Can you work these out from the model? Positions are in its coordinate system, mm. Round coordinates to 2 decimals unless told otherwise and drop trailing zeros. Return JSON: item names as keys, results as strings.
```python
from build123d import *

# Parameters (mm, degrees)
SKETCH_1_W                  = 95
SKETCH_1_H                  = 830
EXTRUDE_1_DEPTH             = 5
HOLE_WIZARD_1_D             = 6.6
HOLE_WIZARD_1_CBORE_D       = 11
HOLE_WIZARD_1_CBORE_DEPTH   = 6.8
HOLE_WIZARD_M8_1_D          = 6.8
HOLE_WIZARD_M8_2_D          = 6.8
HOLE_WIZARD_2_D             = 6.6
HOLE_WIZARD_2_DEPTH         = 10.001
HOLE_WIZARD_2_CBORE_D       = 11
HOLE_WIZARD_2_CBORE_DEPTH   = 6.8
HOLE_WIZARD_M5_1_D          = 4.2
HOLE_WIZARD_1_2_D           = 9
HOLE_WIZARD_1_2_CSINK_D     = 17.6
HOLE_WIZARD_1_2_CSINK_ANGLE = 90


with BuildPart() as part:
    # 草图1 → 凸台-拉伸1 (new body, symmetric)
    with BuildSketch(Plane.XY):
        Rectangle(SKETCH_1_W, SKETCH_1_H)
    extrude(amount=EXTRUDE_1_DEPTH, both=True)

    # Hole Wizard 1 (through all)
    with Locations(Plane(origin=(-20, -365, 5), x_dir=(1, 0, 0), z_dir=(0, 0, 1))):
        with Locations((0, 0), (40, 0), (40, -40), (0, -40), (0, 385), (40, 385), (40, 345), (0, 345), (0, 770), (40, 770), (40, 730), (0, 730)):
            CounterBoreHole(HOLE_WIZARD_1_D / 2, HOLE_WIZARD_1_CBORE_D / 2, HOLE_WIZARD_1_CBORE_DEPTH)

    # M8 螺纹孔1 (through all)
    with Locations(Plane(origin=(0, -400, 5), x_dir=(1, 0, 0), z_dir=(0, 0, 1))):
        with Locations((0, 0), (0, 130)):
            Hole(HOLE_WIZARD_M8_1_D / 2)

    # M8 螺纹孔2 (through all)
    with Locations(Plane(origin=(0, 280, 5), x_dir=(1, 0, 0), z_dir=(0, 0, 1))):
        with Locations((0, 0), (0, -130)):
            Hole(HOLE_WIZARD_M8_2_D / 2)

    # 打孔尺寸(%根据)内六角圆柱头螺钉的类型2
    with Locations(Plane(origin=(41.5, 400, 5), x_dir=(1, 0, 0), z_dir=(0, 0, 1))):
        with Locations((0, 0), (0, -200), (0, -400), (0, -600), (0, -800)):
            hole_wizard_2 = CounterBoreHole(HOLE_WIZARD_2_D / 2, HOLE_WIZARD_2_CBORE_D / 2, HOLE_WIZARD_2_CBORE_DEPTH, depth=HOLE_WIZARD_2_DEPTH)

    # 镜向1: 打孔尺寸(%根据)内六角圆柱头螺钉的类型2 across plane
    add(hole_wizard_2.mirror(Plane(origin=(0, 0, 0), x_dir=(0, 0, 1), z_dir=(1, 0, 0))), mode=Mode.SUBTRACT)

    # M5 螺纹孔1 (through all)
    with Locations(Plane(origin=(0, 395, 5), x_dir=(1, 0, 0), z_dir=(0, 0, 1))):
        with Locations((0, 0), (0, -40)):
            Hole(HOLE_WIZARD_M5_1_D / 2)

    # Hole Wizard 1 2 (through all)
    with Locations(Plane(origin=(-32.5, 24.75, 5), x_dir=(1, 0, 0), z_dir=(0, 0, 1))):
        with Locations((0, 0), (65, 0), (65, -49.5), (0, -49.5), (0, 359.5), (65, 359.5), (65, 310), (0, 310), (0, -359.5), (65, -359.5), (65, -409), (0, -409)):
            CounterSinkHole(HOLE_WIZARD_1_2_D / 2, HOLE_WIZARD_1_2_CSINK_D / 2, counter_sink_angle=HOLE_WIZARD_1_2_CSINK_ANGLE)


solid = part.part
```
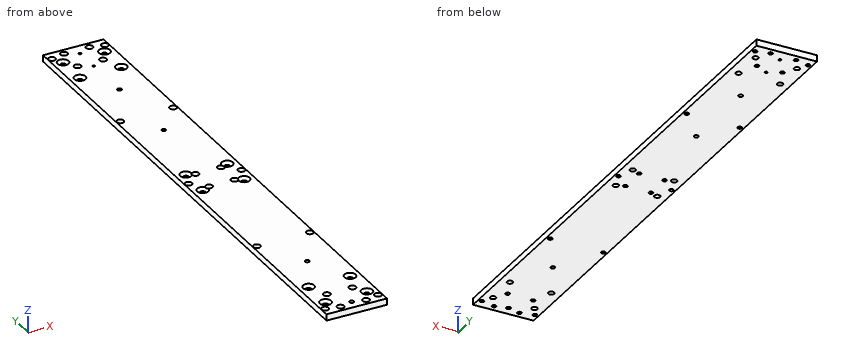
Q1. If I drill on line 1 along X through (y, z) = (203.5, 0); line 2 along X through (y, z) = (29, 3.5), over which ranges is the centre line in solid material (lowest first)?
Results:
{"line 1": "x = -47.5 to -45.74, -37.26 to 37.26, 45.74 to 47.5", "line 2": "x = -47.5 to -38.44, -26.56 to 26.56, 38.44 to 47.5"}
Q2. I'm going to push flat-ended pins straight in: pin 1 Ø9 at (x, y) = (-22, 404) entering from +Z; pin 2 Ø9 at (x, y) = (-41.5, 400) entering from +Z. Where does each tip first touch, or does it pass through?
Results:
{"pin 1": "stops at z = 5", "pin 2": "stops at z = -1.8"}
Q3. Suppose I cut it at A-A, the plane z = 2.75. State how many separate pieces and enclosed holes the cut face has, plus the area to 3 significant figures.
Results:
{"separate pieces": "1", "enclosed holes": "40", "area": "75,000 mm2"}
